```python
from build123d import *

# Parameters (mm, degrees)
EXTRUDE_1_DEPTH     = 2
EXTRUDE_2_DEPTH     = 7
SKETCH_3_W          = 14.5
SKETCH_3_H          = 5.5
CUT_EXTRUDE_1_DEPTH = 2
SKETCH_4_W          = 2
SKETCH_4_H          = 26
EXTRUDE_3_DEPTH     = 1


with BuildPart() as part:
    # 草图1 → 凸台-拉伸1 (new body)
    with BuildSketch(Plane(origin=(0, 0, 0), x_dir=(1, 0, 0), z_dir=(0, 1, 0))):
        with BuildLine():
            Line((14.078397583, 18.946730462), (-15.921602417, 18.946730462))
            ThreePointArc((-15.921602417, 18.946730462), (-10.846789199, 12.197093132), (-9.045997954, 3.946730462))
            ThreePointArc((-9.045997954, 3.946730462), (-10.846789199, -4.303632207), (-15.921602417, -11.053269538))
            Line((-15.921602417, -11.053269538), (14.078397583, -11.053269538))
            Line((14.078397583, -11.053269538), (14.078397583, 18.946730462))
        make_face()
    extrude(amount=EXTRUDE_1_DEPTH)

    # 草图2 → 凸台-拉伸2 (add)
    with BuildSketch(Plane(origin=(0, 2, 0), x_dir=(1, 0, 0), z_dir=(0, 1, 0))):
        with BuildLine():
            Line((14.078397583, 18.946730462), (-15.921602417, 18.946730462))
            ThreePointArc((-15.921602417, 18.946730462), (-14.880689288, 17.982761022), (-13.911474192, 16.946730462))
            Line((-13.911474192, 16.946730462), (12.078397583, 16.946730462))
            Line((12.078397583, 16.946730462), (12.078397583, -9.053269538))
            Line((12.078397583, -9.053269538), (-13.911474192, -9.053269538))
            ThreePointArc((-13.911474192, -9.053269538), (-14.880689288, -10.089300097), (-15.921602417, -11.053269538))
            Line((-15.921602417, -11.053269538), (14.078397583, -11.053269538))
            Line((14.078397583, -11.053269538), (14.078397583, 18.946730462))
        make_face()
    extrude(amount=EXTRUDE_2_DEPTH)

    # 草图3 → 切除-拉伸1 (cut)
    with BuildSketch(Plane.ZY.offset(-12.078397583)):
        with Locations((-3.946730462, 4.75)):
            Rectangle(SKETCH_3_W, SKETCH_3_H)
    extrude(amount=-CUT_EXTRUDE_1_DEPTH, mode=Mode.SUBTRACT)

    # 草图4 → 凸台-拉伸3 (add)
    with BuildSketch(Plane(origin=(0, 2, 0), x_dir=(1, 0, 0), z_dir=(0, 1, 0))):
        with Locations((3.578397583, 3.946730462)):
            Rectangle(SKETCH_4_W, SKETCH_4_H)
    extrude(amount=EXTRUDE_3_DEPTH)


solid = part.part
```
Input: part model. Units: mm. Frame: model coordinates. A direction names the side the tool comes from. Give positions to 0.01 mm unless a question says otherwise; leave off trailing zeros. Write each loop counter-clockwise with the first axis right and the second up, starting at its lowest first coordinate (ties: lowest second). Pieces come first, ordered by that corner, then holes. Notation, with made-up numbers: (10, -38) - (19, -38) arc R21 cw to (19, -30) - close; hole circle Ø3 at (42.5, 48). An arc over 180 degrees is marked (long way). Write item = value, one per line. Start each with the question number.
1) Cut plane B-B (z = -3.5). Return loops of the section in (x, y).
2) Pin query (flat end, axial travel): pin 1 (0.8 mm diameter, centred on y = 2.5, z = -8.5, fed in from +X); pin 2 (4 mm diameter, centred on x = 0.5, z = -5.5, fed in from +Y); pin 3 (3.5 mm diameter, centred on y = 6, z = 1, fed in from -X). Return the tip coordinate at first contact, or that it passes through.
3) Cut plane D-D (y = 2.5). Return loops of the section in (x, z), and give its area (3 significant figures).
4) Cut plane A-A (y = 6.75). Return loops of the section in (x, z), and give its area (3 significant figures).
5) Reachability of faces 4 (the face through (2.578, 2.5, -3.8)), 5 (the face through (9, 2, -4)), 6 (the face through (13, 7.5, -4)), 7 (the face through (4.578, 2.5, -3.8)), 8 (the face through (13, 5, -11.197)) from +Z, -Z, +X, -X, +Y, -Y: full face, straight path, thin tool, end or side. Return the list, or none.
6) Material intervals for L1, parallel to Z at x = 0.5, y = 2.25; L2, parallel to Z at x = 12.25, y = 5.5; L3, parallel to Y at x = 12.75, z = -5.5, sorted ascending. Write a range as [from, to].
7) Cut plane C-C (x = 3). Return loops of the section in (y, z).
8) Draft query along Y for faces 1 (the face through (-4, 2, -4)), 2 (the face through (12.078, 8, -4)), 3 (the face through (13, 5, 3.303)). Return one class per face: pulls with the +Y half, pulls with the -Y half, needs draft (parallel to the pull), parting line crosses it, or undercut.
Answers follow:
q1.outline = (-9.05, 0) - (14.08, 0) - (14.08, 2) - (4.58, 2) - (4.58, 3) - (2.58, 3) - (2.58, 2) - (-9.05, 2) - close; (12.08, 7.5) - (14.08, 7.5) - (14.08, 9) - (12.08, 9) - close
q2.pin_1 = 4.58
q2.pin_2 = 2
q2.pin_3 = 12.08
q3.outline = (-15.92, -18.95) - (14.08, -18.95) - (14.08, -11.2) - (12.08, -11.2) - (12.08, -16.95) - (4.58, -16.95) - (4.58, 9.05) - (12.08, 9.05) - (12.08, 3.3) - (14.08, 3.3) - (14.08, 11.05) - (-15.92, 11.05) arc R19.8 cw to (-13.91, 9.05) - (2.58, 9.05) - (2.58, -16.95) - (-13.91, -16.95) arc R19.8 cw to start
q3.area = 191 mm^2
q4.outline = (-15.92, -18.95) - (14.08, -18.95) - (14.08, -11.2) - (12.08, -11.2) - (12.08, -16.95) - (-13.91, -16.95) arc R19.8 cw to start; (-15.92, 11.05) arc R19.8 cw to (-13.91, 9.05) - (12.08, 9.05) - (12.08, 3.3) - (14.08, 3.3) - (14.08, 11.05) - close
q4.area = 139 mm^2
q5.face_4 = -X, +Y
q5.face_5 = none
q5.face_6 = +X, -X
q5.face_7 = +Y
q5.face_8 = +X
q6.L1 = [-18.95, -16.95], [9.05, 11.05]
q6.L2 = [-18.95, -11.2], [3.3, 11.05]
q6.L3 = [0, 2], [7.5, 9]
q7.outline = (0, -18.95) - (9, -18.95) - (9, -16.95) - (3, -16.95) - (3, 9.05) - (9, 9.05) - (9, 11.05) - (0, 11.05) - close
q8.face_1 = pulls with the +Y half
q8.face_2 = needs draft
q8.face_3 = undercut
